from build123d import *

# Parameters (mm, degrees)
F1_DEPTH = 1.27
F2_R     = 0.762
F3_DEPTH = 0.635
F4_SIZE  = 0.63499


# Not quite as in the source:
# - a fillet or chamfer is up to 0.001 mm smaller than in the source, because OpenCascade refuses the exact size


with BuildPart() as f1:
    # F0 (on Front) → F1 (new body, symmetric)
    with BuildSketch(Plane.XZ):
        Polygon((-30.9530049562, -3.3370526507), (-30.1719289273, -1.8979058368), (-34.4893708825, 0), (-35.9563070381, -3.3370526507), align=None)
        Polygon((-30.1719289273, -4.7761994647), (-30.9530049562, -3.3370526507), (-35.9563070381, -3.3370526507), (-34.4893708825, -6.6741053015), align=None)
        Polygon((-1.278280112, -3.4174603466), (0, 0), (-30.1719289273, -1.8979058368), (-30.9530049562, -3.3370526507), align=None)
        Polygon((0, -6.6741053015), (-1.278280112, -3.4174603466), (-30.9530049562, -3.3370526507), (-30.1719289273, -4.7761994647), align=None)
    extrude(amount=F1_DEPTH, both=True)

    # F2
    f2_edges = [f1.edges().sort_by_distance(p)[0] for p in [
        (-15.085964, -1.27, -0.948953),
        (-15.085964, 1.27, -0.948953),
        (-15.085964, 1.27, -5.725152),
        (-15.085964, -1.27, -5.725152),
    ]]
    fillet(f2_edges, radius=F2_R)

    # F0 (on Front) → F3 (join, symmetric)
    with BuildSketch(Plane.XZ):
        Polygon((-1.278280112, -3.4174603466), (0, 0), (-30.1719289273, -1.8979058368), (-30.9530049562, -3.3370526507), align=None)
        Polygon((3.6480247509, 4.5782560483), (0, 0), (-1.278280112, -3.4174603466), (105.1078885794, -3.3370526507), (75.8452340961, 0), (9.3937172488, 0), align=None)
        Polygon((-30.9530049562, -3.3370526507), (-30.1719289273, -1.8979058368), (-34.4893708825, 0), (-35.9563070381, -3.3370526507), align=None)
        Polygon((105.1078885794, -3.3370526507), (-1.278280112, -3.4174603466), (0, -6.6741053015), (3.6480247509, -11.2523613498), (9.3937172488, -6.6741053015), (75.8452340961, -6.6741053015), align=None)
        Polygon((0, -6.6741053015), (-1.278280112, -3.4174603466), (-30.9530049562, -3.3370526507), (-30.1719289273, -4.7761994647), align=None)
        Polygon((-30.1719289273, -4.7761994647), (-30.9530049562, -3.3370526507), (-35.9563070381, -3.3370526507), (-34.4893708825, -6.6741053015), align=None)
    extrude(amount=F3_DEPTH, both=True)

    # F4 (size 0.635 in the source; OpenCascade refuses exactly that, so slightly less here)
    f4_edges = [f1.edges().sort_by_distance(p)[0] for p in [
        (42.619476, -0.635, -6.674105),
        (42.619476, 0.635, -6.674105),
        (42.619476, -0.635, 0),
        (42.619476, 0.635, 0),
        (90.476561, -0.635, -1.668526),
        (90.476561, 0.635, -1.668526),
        (90.476561, -0.635, -5.005579),
        (90.476561, 0.635, -5.005579),
    ]]
    chamfer(f4_edges, length=F4_SIZE)


solid = f1.part
The listing builds one solid part. Answer for the finished solid, in the listing's coordinates (mm). A direction names the side the tool comes from. Give positions to 0.01 mm unless a question says otherwise; leave off trailing zeros. Loops run counter-clockwise (first coordinate to the right, second up) from the corner with the lowest first, then second, coordinate; pieces in that order, holes last. Notation, with made-up numbers: M 84.25,27 L 124.25,27 A27 ccw 124.25,44 Z; hole C -10,21.5 d11. An arc over 180 degrees is marked long. Answer as CSV lines item,"result".
Item 1: Straight lines are drawn through the part: line 1 along Y through (x, z) = (30.5, -1.5) (3 decimals); line 2 along Z through (x, y) = (91.5, -0.15); line 3 along Z through (x, y) = (-26, 0.8). For each, find the intervals that lie inside material, in ascending order. Write a range as [from, to].
Values follow:
line 1,"y = [-0.635, 0.635]"
line 2,"z = [-4.74, -1.94]"
line 3,"z = [-4.98, -1.69]"
Item 2: The part is cut by section B-B (z = -8.25). Give the vertices of the cut face in (x, y) (3 decimals).
Values follow:
outline,"M 1.256,-0.635 L 7.416,-0.635 L 7.416,0.635 L 1.256,0.635 Z"
Item 3: Which of the six approach directions +Z, -Z, +X, -X, +Y, -Y give full straight-line access (tool end or side, diameter ignored) to faces 1 (the cylindrical face through (-14.851, 1.085, -5.475)), 2 (the cylindrical face through (-15.27, -1.09, -1.23)), 3 (the flat face through (90.24, 0.32, -4.71))?
Values follow:
face 1,"-Z, +Y"
face 2,"+Z, -Y"
face 3,"-Z, +X, +Y"
Item 4: The part is cut by section D-D (z = 3). Give the vertices of the cut face in (x, y) (3 decimals).
Values follow:
outline,"M 2.39,-0.635 L 5.629,-0.635 L 5.629,0.635 L 2.39,0.635 Z"
Item 5: The mould has two halves that part along X. Classify faces 4 (the cylindrical face through (-15.27, 1.09, -1.23)), 5 (the flat face through (-18, 1.27, -3)), 6 (the flat face through (90.64, -0.32, -2.01)): released by +X, released by -X, zero draft, split by the parting line, or undercut.
Values follow:
face 4,"undercut"
face 5,"zero draft"
face 6,"released by +X"
Item 6: Given pin 1 Ø1 at (y, z) = (0.5, -5.5) entering from -X; pin 2 Ø4.5 at (x, z) = (26.5, -1) entering from +Y (3 decimals); pin 3 Ø8 at (x, z) = (42, -7) entering from -Y (3 decimals), each flat-ended and moving along its own axis, determine where each tip first touches the part or whether it passes through.
Values follow:
pin 1,"stops at x = -35.23"
pin 2,"stops at y = 0.635"
pin 3,"stops at y = -0.635"
